The drawing under review shows one solid part. Ordinate dimensions are in mm from its lowest x, y, z. A direction names the side the tool comes from. Round coordinates to 2 decimals unless told otherwise and drop trailing zeros. Loops run counter-clockwise (first coordinate to the right, second up) from the corner with the lowest first, then second, coordinate; pieces in that order, holes last. Notation, with made-up numbers: M 39.25,46.25 L 98.25,46.25 A8 cw 98.25,58.25 Z; hole C 50,-12.75 d5. An arc over 180 degrees is marked long. Use a Markdown table: item, result.
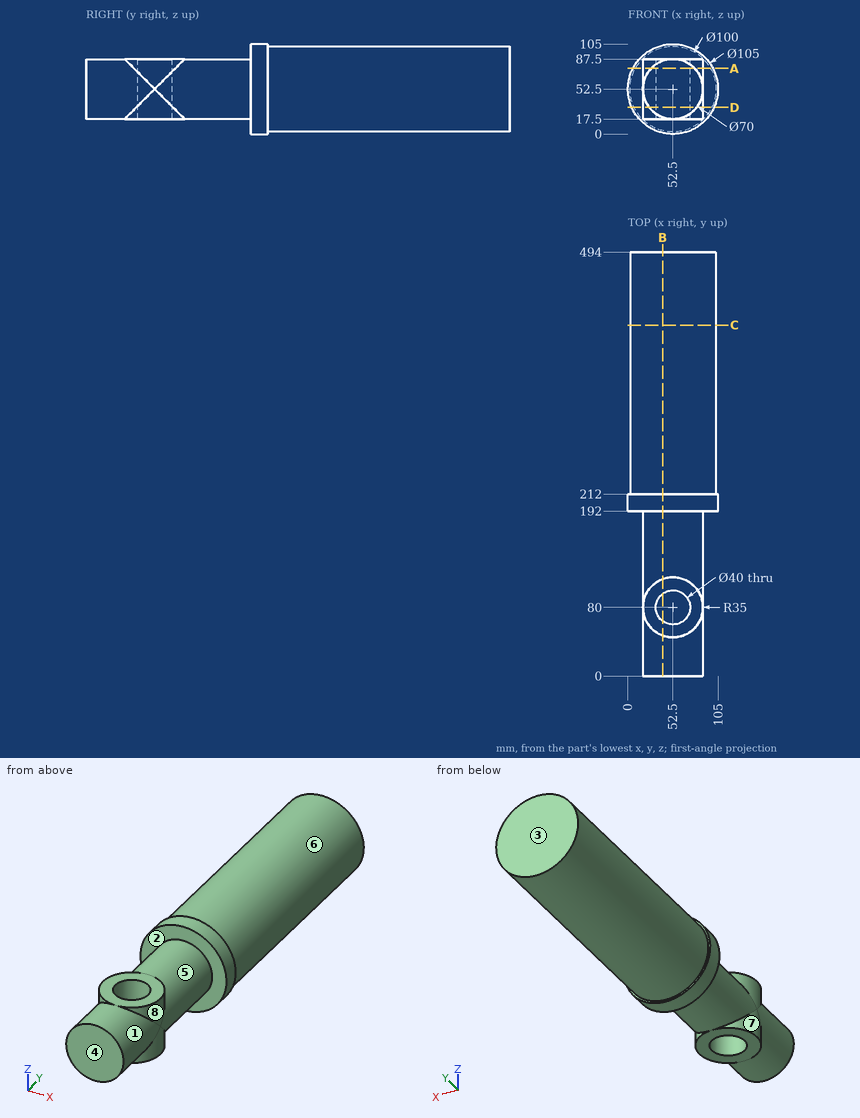
1. Wall thickness on line 1 along Y through (x, z) = (52, 57); line 2 along X through (y, z) = (80, 45); line 3 along Y through (x, z) = (5.5, 43.5): over which ranges is each line inside the solid? List them lowest first. Write a range as from..to.
Check values:
| item | result |
|---|---|
| line 1 | y = 0..60.01, 99.99..494 |
| line 2 | x = 17.5..32.5, 72.5..87.5 |
| line 3 | y = 192..494 |
2. Insertion check: pin 1 (1 mm diameter, centred on x = 61, y = 165, fed in from -Z); pin 2 (1 mm diameter, centred on x = 73.5, y = 70, fed in from -Z); pin 3 (1 mm diameter, centred on y = 359.5, z = 85.5, fed in from -X). Each pin has a flat end and moves straight along its axis. Give the tip position at first contact, or say it passes through.
Check values:
| item | result |
|---|---|
| pin 1 | stops at z = 18.43 |
| pin 2 | stops at z = 17.5 |
| pin 3 | stops at x = 14.5 |
3. The part is to be moulded in two halves that separate along Y. For the marked faces 1, 2, 3 and 4, say which applies: pulls with the +Y half, pulls with the -Y half, needs draft (parallel to the pull), parting line crosses it, or undercut.
Check values:
| item | result |
|---|---|
| face 1 | needs draft |
| face 2 | undercut |
| face 3 | pulls with the +Y half |
| face 4 | pulls with the -Y half |
4. Take a section at B-B on x = 40.5. Give the boundary of the cut face in (y, z).
Check values:
| item | result |
|---|---|
| outline | M 0,19.62 L 47.12,19.62 L 47.12,17.5 L 64,17.5 L 64,87.5 L 47.12,87.5 L 47.12,85.38 L 0,85.38 Z; M 96,17.5 L 112.88,17.5 L 112.88,19.62 L 192,19.62 L 192,1.39 L 212,1.39 L 212,3.96 L 494,3.96 L 494,101.04 L 212,101.04 L 212,103.61 L 192,103.61 L 192,85.38 L 112.88,85.38 L 112.88,87.5 L 96,87.5 Z |
5. Take a section at D-D on z = 31. Give the boundary of the cut face in (x, y).
Check values:
| item | result |
|---|---|
| outline | M 4.6,192 L 24.88,192 L 24.88,101.5 A35 ccw 24.88,58.5 L 24.88,0 L 80.12,0 L 80.12,58.5 A35 ccw 80.12,101.5 L 80.12,192 L 100.4,192 L 100.4,212 L 97.64,212 L 97.64,494 L 7.36,494 L 7.36,212 L 4.6,212 Z; hole C 52.5,80 d40 |
6. Machinability: for the marked faces 5, 6, 7 and 8, which of the approach directions +Z, -Z, +X, -X, +Y, -Y give a long, thin tool a straight path to every point of the face, cutting with its end or side? Answer none if there is none.
Check values:
| item | result |
|---|---|
| face 5 | none |
| face 6 | +Y |
| face 7 | -Z, -X |
| face 8 | +Z, +X |
7. Take a section at C-C on y = 409. Give the boundary of the cut face in (x, z).
Check values:
| item | result |
|---|---|
| outline | C 52.5,52.5 d100 |
8. Take a section at A-A on z = 76.5. Give the boundary of the cut face in (x, y).
Check values:
| item | result |
|---|---|
| outline | M 5.81,192 L 27.02,192 L 27.02,104 A35 ccw 27.02,56 L 27.02,0 L 77.98,0 L 77.98,56 A35 ccw 77.98,104 L 77.98,192 L 99.19,192 L 99.19,212 L 96.36,212 L 96.36,494 L 8.64,494 L 8.64,212 L 5.81,212 Z; hole C 52.5,80 d40 |
